CAD build for the part. Positions are in the model's coordinates, mm. A direction names the side the tool comes from. Coordinates: 2 decimals unless noted, no trailing zeros. Loops run counter-clockwise (first coordinate to the right, second up) from the corner with the lowest first, then second, coordinate; pieces in that order, holes last. Notation, with made-up numbers: (63.25, 67.25) - (80.25, 67.25) arc R32 cw to (80.25, 102.25) - close; hole circle Ø11 at (-14.75, 8.5). An arc over 180 degrees is marked (long way). Put each result on its own line as item: value.
Autodesk Inventor part; units mm, degrees
ref_plane "Work Plane1" through (40, 0, 0) normal (1, 0, 0) x (0, 0, -1)
ref_plane "YZ Plane" through (0, 0, 0) normal (1, 0, 0) x (0, 1, 0)
ref_plane "XZ Plane" through (0, 0, 0) normal (0, 1, 0) x (-1, 0, 0)
sketch "Sketch1" plane through (0, 0, 0) normal (1, 0, 0) x (0, 1, 0)
  line L0 (-15, 40) -> (15, 40)
  line L1 (15, 40) -> (15, -40)
  line L2 (15, -40) -> (-15, -40)
  line L3 (-15, -40) -> (-15, 40)
  line L4 (-15, 40) -> (15, -40) construction
  line L5 (15, 40) -> (-15, -40) construction
  point P0 (0, 0)
  dimension "d0" = 30
  dimension "d1" = 80
extrude "Extrusion1" add sketch "Sketch1" along normal blind 80
sketch "Sketch2" plane through (80, 0, 0) normal (1, 0, 0) x (0, 0, -1)
  line L0 (-40, 15) -> (-40, -15)
  line L1 (-40, 0) -> (40, 0)
  line L2 (40, -15) -> (40, 15)
  line L3 (40, 15) -> (-40, 15)
  line L4 (0, 15) -> (0, -15)
  line L5 (-40, -15) -> (40, -15)
  point P0 (0, 0)
  point P1 (-19, 0)
  point P2 (19, 0)
  dimension "d4" = 19
hole "Hole1" at (80, 0, 19) at (80, 0, -19) direction (-1, 0, 0) diameter 13.835 depth 40 tip angle 118
ref_plane "Work Plane1" through (40, 0, 0) normal (1, 0, 0) x (0, 0, -1)
mirror "Mirror1" about plane through (40, 0, 0) normal (1, 0, 0) of "Hole1"
sketch "Sketch9" plane through (0, -15, -40) normal (0, 0, -1) x (-1, 0, 0)
  line L0 (0, 0) -> (-80, 0)
  line L1 (0, 30) -> (-80, 30)
  line L2 (-80, 0) -> (-80, 30)
  line L3 (-20, 30) -> (-10, 30)
  line L4 (-10, 30) -> (-10, 0)
  line L5 (-10, 0) -> (-20, 0)
  line L6 (-20, 0) -> (-20, 30)
  line L7 (0, 30) -> (0, 0)
  line L8 (-60, 30) -> (-70, 30)
  line L9 (-70, 30) -> (-70, 0)
  line L10 (-70, 0) -> (-60, 0)
  line L11 (-60, 0) -> (-60, 30)
  dimension "d78" = 10
  dimension "d79" = 10
  dimension "d80" = 10
  dimension "d81" = 10
extrude "Extrusion4" add sketch "Sketch9" along normal blind 40 contours L0 L6 L1 L4 | L0 L9 L1 L11
hole "Hole6" at (70, 0, -65) direction (-1, 0, 0) diameter 13.5 end through all
fillet "Fillet12" radius 10 4 edges at (70, 0, -40) (60, 0, -40) (20, 0, -40) (10, 0, -40)
fillet "Fillet14" radius 2 4 edges at (15, 15, -80) (15, -15, -80) (65, 15, -80) (65, -15, -80)
fillet "Fillet15" radius 2 2 edges at (40, 15, 40) (40, -15, 40)
properties part number "Profile_Middle_05"
Q1. Slice it at D-D, the plane z = -19. Give the cut face in (x, y), then the cut area to 3 significant figures.
Determined:
outline: (0, -15) - (80, -15) - (80, -6.92) - (0, -6.92) - close; (0, 6.92) - (80, 6.92) - (80, 15) - (0, 15) - close
area: 1,290 mm2
Q2. Pin check, flat tips, straight feed: pin 1 Ø1.5 at (x, y) = (43, 3.5) entering from -Z; pin 2 Ø10 at (y, z) = (2.5, -49.5) entering from +X; pin 3 Ø17.5 at (y, z) = (0, -65) entering from +X. Stop position of each tip, or through.
Determined:
pin 1: z = -40
pin 2: x = 71.65
pin 3: x = 70
Q3. Slice it at C-C, the plane x = 43.5. Give the cut face in (y, z) (1 decimal), then the cut area to 3 significant figures.
Determined:
outline: (-15, -40) - (15, -40) - (15, 38) arc R2 ccw to (13, 40) - (-13, 40) arc R2 ccw to (-15, 38) - close; hole circle Ø13.8 at (0, -19); hole circle Ø13.8 at (0, 19)
area: 2,100 mm2
Q4. Slice it at B-B, the plane z = -65. Give the cut face in (x, y).
Determined:
outline: (10, -15) - (20, -15) - (20, -6.75) - (10, -6.75) - close; (10, 6.75) - (20, 6.75) - (20, 15) - (10, 15) - close; (60, -15) - (70, -15) - (70, -6.75) - (60, -6.75) - close; (60, 6.75) - (70, 6.75) - (70, 15) - (60, 15) - close
Q5. Wall check: L1, parallel to Z at x = 65.5, y = 0; L2, parallel to Z at x = 31.5, y = 0; L3, parallel to Y at x = 52, z = -19. Give the ranges that are in metal, low to high. Write a range as from..to.
Determined:
L1: -80..-71.75, -58.25..-25.92, -12.08..12.08, 25.92..40
L2: -40..-25.92, -12.08..12.08, 25.92..40
L3: -15..-6.92, 6.92..15
Q6. Slice it at A-A, the plane y = 0. State how many separate pieces and enclosed holes the cut face has, then the cut area to 3 significant figures.
Determined:
separate pieces: 5
enclosed holes: 0
area: 4,800 mm2
Q7. Tool access for faces 1 (the cylindrical face through (14.93, -0.297, -58.257)), 2 (the flat face through (20, -7, -65)), 3 (the flat face through (10, 7, -65)), 4 (the flat face through (15, 0, -80)), 5 (the flat face through (70, 7, -65)): list every direction of +Z, -Z, +X, -X, +Y, -Y with a clear straight run to the whole face (end or side of a thin tool).
Determined:
face 1: +X, -X
face 2: -Z, +Y, -Y
face 3: -Z, -X, +Y, -Y
face 4: -Z, +X, -X, +Y, -Y
face 5: -Z, +X, +Y, -Y
Q8. Mould opens along Z. For faces 6 (the cylindrical face through (64.93, -0.297, -58.257)), 7 (the flat face through (80, 0, 1)), 8 (the flat face through (39, 0, 40)) say: +Z half, -Z half, draft (parallel to the pull), parting line (faces both ways), or undercut.
Determined:
face 6: undercut
face 7: draft
face 8: +Z half
